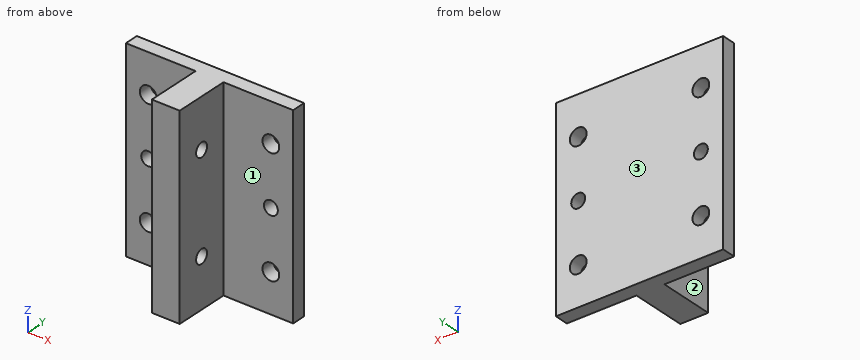
```python
from build123d import *

# Parameters (mm, degrees)
F0_W     = 60
F0_H     = 70
F0_R     = 3
F0_R_2   = 2.5
F1_DEPTH = 5
F2_W     = 10
F2_H     = 70
F3_DEPTH = 20
F5_D     = 5
F5_DEPTH = 40


with BuildPart() as f1:
    # F0 (on Front) → F1 (new body)
    with BuildSketch(Plane.XZ):
        Rectangle(F0_W, F0_H)
        with Locations((-22, -21)):
            Circle(F0_R, mode=Mode.SUBTRACT)
        with Locations((22, -21)):
            Circle(F0_R, mode=Mode.SUBTRACT)
        with Locations((-22, 0)):
            Circle(F0_R_2, mode=Mode.SUBTRACT)
        with Locations((-22, 21)):
            Circle(F0_R, mode=Mode.SUBTRACT)
        with Locations((22, 0)):
            Circle(F0_R_2, mode=Mode.SUBTRACT)
        with Locations((22, 21)):
            Circle(F0_R, mode=Mode.SUBTRACT)
    extrude(amount=F1_DEPTH)

    # F2 (on face) → F3 (join)
    with BuildSketch(Plane.XZ.offset(5)):
        Rectangle(F2_W, F2_H)
    extrude(amount=F3_DEPTH)

    # F5
    with Locations(Plane.YZ.offset(5)):
        with Locations((-15, 17.5), (-15, -17.5)):
            Hole(F5_D / 2, depth=F5_DEPTH)


solid = f1.part
```
Check sheet for the modelled part. Datum: model origin and axes. Units: mm. Face numbers are marked on the shaded views. A direction names the side the tool comes from. Round coordinates to 2 decimals unless told otherwise and drop trailing zeros. Loops run counter-clockwise (first coordinate to the right, second up) from the corner with the lowest first, then second, coordinate; pieces in that order, holes last. Notation, with made-up numbers: (67, 43) - (102, 43) arc R13 ccw to (102, 61) - close; hole circle Ø5 at (33, 80.5). An arc over 180 degrees is marked (long way). Write item = value, one per line. Start each with the question number.
Q1. Section check D-D (z = 5). Record the boundary of the cut face in (x, y), plus the area to 3 significant figures.
Q2. Access from +Z, -Z, +X, -X, +Y, -Y to the whole of each face (thin tool, end or side, straight path). Record for the marked faces 1, 2 and 3.
Q3. Section check A-A (z = -21). Record the boundary of the cut face in (x, y), plus the area to 3 significant figures.
Q4. Thickness scan on L1, parallel to Z at x = 0.25, y = -15; L2, parallel to Z at x = 22, y = -3.4; L3, parallel to Z at x = -1, y = -16.25. Record the ranges inside material, lowest first.
Q5. Depth check by flat-ended pin: P1, Ø6, axis at y = -16.5, z = 16.5, coming from the +X side; P2, Ø3, axis at y = -12, z = -20, coming from the -X side; P3, Ø9.5, axis at x = -22, z = -21, coming from the -Y side. Enter the tip coordinate at first touch or a pass-through.
Q6. Section check C-C (y = -15). Record the boundary of the cut face in (x, z).
Q7. Section check B-B (x = 22). Record the boundary of the cut face in (y, z).
Derived:
q1.outline = (-30, -5) - (-5, -5) - (-5, -25) - (5, -25) - (5, -5) - (30, -5) - (30, 0) - (-30, 0) - close
q1.area = 500 mm^2
q2.face_1 = +Z, -Z, +X, -Y
q2.face_2 = +Z, -Z, -X, -Y
q2.face_3 = +Z, -Z, +X, -X, +Y
q3.outline = (-30, -5) - (-25, -5) - (-25, 0) - (-30, 0) - close; (-19, -5) - (-5, -5) - (-5, -25) - (5, -25) - (5, -5) - (19, -5) - (19, 0) - (-19, 0) - close; (25, -5) - (30, -5) - (30, 0) - (25, 0) - close
q3.area = 440 mm^2
q4.L1 = -35 to -20, -15 to 15, 20 to 35
q4.L2 = -35 to -24, -18 to -2.5, 2.5 to 18, 24 to 35
q4.L3 = -35 to -19.67, -15.33 to 15.33, 19.67 to 35
q5.P1 = 5
q5.P2 = -5
q5.P3 = -5
q6.outline = (-5, -35) - (5, -35) - (5, -20) - (-5, -20) - close; (-5, -15) - (5, -15) - (5, 15) - (-5, 15) - close; (-5, 20) - (5, 20) - (5, 35) - (-5, 35) - close
q7.outline = (-5, -35) - (0, -35) - (0, -24) - (-5, -24) - close; (-5, -18) - (0, -18) - (0, -2.5) - (-5, -2.5) - close; (-5, 2.5) - (0, 2.5) - (0, 18) - (-5, 18) - close; (-5, 24) - (0, 24) - (0, 35) - (-5, 35) - close
